Geometry check sheet. Reference: the model listing, model coordinates, mm. A direction names the side the tool comes from. Give positions to 0.01 mm unless a question says otherwise; leave off trailing zeros. Order: outer loops, then holes, each group sorted by start corner. A loop starts at its lowest first (then second) coordinate and runs counter-clockwise, first axis right, second up. Notation, with made-up numbers: M -7,-28.5 L 30,-28.5 A22 ccw 30,0.5 Z; hole C -30.5,61 d9. An arc over 180 degrees is marked long. One line per question, with ' | ' between items. Start each with the question number.
from build123d import *

# Parameters (mm, degrees)
F2_SIZE = 2.54
F3_R    = 3.175


with BuildPart() as f1:
    # F0 (on Front) → F1 (revolve)
    with BuildSketch(Plane.XZ):
        Polygon((8.6614, 13.000173), (0, 13.000173), (0, -12.399827), (30.1625, -12.399827), (30.1625, -8.589827), (19.05, -0.971779), (15.875, -0.971779), (8.6614, 0.300173), align=None)
    revolve(axis=Axis((0, 0, 1.824711), (0, 0, -1)))

    # F2
    f2_edges = [f1.edges().sort_by_distance(p)[0] for p in [
        (-8.6614, 0, 13.000173),
    ]]
    chamfer(f2_edges, length=F2_SIZE)

    # F3
    f3_edges = [f1.edges().sort_by_distance(p)[0] for p in [
        (-30.1625, 0, -12.399827),
    ]]
    fillet(f3_edges, radius=F3_R)


solid = f1.part
Item 1: Cross-section at D-D, the plane z = -7. Record the cut outline in (x, y).
Item 2: Set-up check for faces 1 (the flat face through (0, 0, 13)), 2 (the cylindrical face through (3.997, 7.684, 5.451)): record each of +Z, -Z, +X, -X, +Y, -Y from which the full face is reachable in a straight line by a thin tool's end or side.
Item 3: Material ranges on line 1 along Z through (x, y) = (-17.5, -4); line 2 along X through (y, z) = (-10.5, -4); line 3 along Z through (x, y) = (-25.5, 7), recorded low to high.
Item 4: Cross-section at C-C, the plane z = 4. Record the cut outline in (x, y), plus the area to 3 significant figures.
Item 5: Depth check by flat-ended pin: pin 1 (3 mm diameter, centred on x = 8, z = 4.5, fed in from -Y); pin 2 (4 mm diameter, centred on x = 14.5, y = 3, fed in from +Z); pin 3 (5 mm diameter, centred on y = -19.5, z = -9.5, fed in from -X); pin 4 (6 mm diameter, centred on x = -18, z = 4.5, fed in from +Y). Enter the tip coordinate at first touch or a pass-through.
Outcome:
1) outline: C 0,0 d55.69
2) face 1: +Z, +X, -X, +Y, -Y | face 2: +Z
3) line 1: z = -12.4 to -0.97 | line 2: x = -20.99 to 20.99 | line 3: z = -12.4 to -6.04
4) outline: C 0,0 d17.32 | area: 236 mm²
5) pin 1: stops at y = -5.72 | pin 2: stops at z = -0.43 | pin 3: stops at x = -24.91 | pin 4: passes through
